Source: CAD feature listing. Evaluate the final solid. Frame: model axes, mm. A direction names the side the tool comes from. Give positions to 0.01 mm unless a question says otherwise; leave off trailing zeros. Write each loop counter-clockwise with the first axis right and the second up, starting at its lowest first coordinate (ties: lowest second). Pieces come first, ordered by that corner, then holes.
```python
from build123d import *

# Parameters (mm, degrees)
F0_W        = 3.9569679648
F0_H        = 9.3060303107
F0_R        = 0.75
F1_DEPTH    = 2
F2_R        = 3.6
F3_DEPTH    = 25
F4_T1_DEPTH = 2
F4_T3_DEPTH = 12


# Not quite as in the source:
# - a fillet or chamfer that OpenCascade refuses, or shapes differently, is made with other operations: its cross-section is extruded or revolved along the edge and cut away or added


with BuildPart() as f1:
    # F0 (on Top) → F1 (new body)
    with BuildSketch(Plane.XY):
        with Locations((-9.7150150687, 6.8534435891)):
            Rectangle(F0_W, F0_H)
        with Locations((-9.7150150687, 7.7160103247)):
            Circle(F0_R, mode=Mode.SUBTRACT)
        with Locations((-9.7150150687, 9.6662240103)):
            Circle(F0_R, mode=Mode.SUBTRACT)
        with BuildLine():
            ThreePointArc((-3.4285871837, -2.0602887962), (-3.9991430252, 0.0827953119), (-3.3403764321, 2.2004284337))
            Line((-3.3403764321, 2.2004284337), (-7.7365310863, 2.2004284337))
            Line((-7.7365310863, 2.2004284337), (-11.693499051, 2.2004284337))
            Line((-11.693499051, 2.2004284337), (-11.693499051, -2.0602887962))
            Line((-11.693499051, -2.0602887962), (-3.4285871837, -2.0602887962))
        make_face()
        with Locations((-9.7150150687, 0)):
            Circle(F0_R, mode=Mode.SUBTRACT)
        with BuildLine():
            Line((3.3403764321, -2.0602887962), (3.3403764321, 2.2004284337))
            ThreePointArc((3.3403764321, 2.2004284337), (0, 4), (-3.3403764321, 2.2004284337))
            Line((-3.3403764321, 2.2004284337), (-3.3403764321, -2.0602887962))
            Line((-3.3403764321, -2.0602887962), (-3.4285871837, -2.0602887962))
            ThreePointArc((-3.4285871837, -2.0602887962), (0, -4), (3.4285871837, -2.0602887962))
            Line((3.4285871837, -2.0602887962), (3.3403764321, -2.0602887962))
        make_face()
        with BuildLine():
            ThreePointArc((3.3403764321, 2.2004284337), (3.8315470588, 1.1485848405), (4, 0))
            ThreePointArc((4, 0), (3.8545005341, -1.06903023), (3.4285871837, -2.0602887962))
            Line((3.4285871837, -2.0602887962), (11.693499051, -2.0602887962))
            Line((11.693499051, -2.0602887962), (11.693499051, 2.2004284337))
            Line((11.693499051, 2.2004284337), (7.7365310863, 2.2004284337))
            Line((7.7365310863, 2.2004284337), (3.3403764321, 2.2004284337))
        make_face()
        with Locations((9.7150150687, 0)):
            Circle(F0_R, mode=Mode.SUBTRACT)
        with Locations((9.7150150687, 6.8534435891)):
            Rectangle(F0_W, F0_H)
        with Locations((9.7150150687, 7.7160103247)):
            Circle(F0_R, mode=Mode.SUBTRACT)
        with Locations((9.7150150687, 9.6662240103)):
            Circle(F0_R, mode=Mode.SUBTRACT)
        with BuildLine():
            Line((-3.3403764321, -2.0602887962), (-3.3403764321, 2.2004284337))
            ThreePointArc((-3.3403764321, 2.2004284337), (-3.9991430252, 0.0827953119), (-3.4285871837, -2.0602887962))
            Line((-3.4285871837, -2.0602887962), (-3.3403764321, -2.0602887962))
        make_face()
        with BuildLine():
            ThreePointArc((3.4285871837, -2.0602887962), (3.8545005341, -1.06903023), (4, 0))
            ThreePointArc((4, 0), (3.8315470588, 1.1485848405), (3.3403764321, 2.2004284337))
            Line((3.3403764321, 2.2004284337), (3.3403764321, -2.0602887962))
            Line((3.3403764321, -2.0602887962), (3.4285871837, -2.0602887962))
        make_face()
    extrude(amount=F1_DEPTH)

    # F2 (on face) → F3 (cut)
    with BuildSketch(Plane.XY.offset(2)):
        Circle(F2_R)
    extrude(amount=-F3_DEPTH, mode=Mode.SUBTRACT)

    # F4: fillet of radius 2 on 8 edges, made by hand

    # F4_s2 → F4_t1 (join)
    with BuildSketch(Plane.XY):
        with BuildLine():
            ThreePointArc((-7.7365310863, 4.2004284337), (-7.1507446486, 2.7862148714), (-5.7365310863, 2.2004284337))
            Line((-5.7365310863, 2.2004284337), (-7.7365310863, 2.2004284337))
            Line((-7.7365310863, 2.2004284337), (-7.7365310863, 4.2004284337))
        make_face()
        with BuildLine():
            ThreePointArc((5.7365310863, 2.2004284337), (7.1507446486, 2.7862148714), (7.7365310863, 4.2004284337))
            Line((7.7365310863, 4.2004284337), (7.7365310863, 2.2004284337))
            Line((7.7365310863, 2.2004284337), (5.7365310863, 2.2004284337))
        make_face()
    extrude(amount=F4_T1_DEPTH)

    # F4_s4 → F4_t3 (cut)
    with BuildSketch(Plane.XY.offset(-5)):
        with BuildLine():
            ThreePointArc((9.693499051, 11.5064587444), (11.1077126134, 10.9206723068), (11.693499051, 9.5064587444))
            Line((11.693499051, 9.5064587444), (11.693499051, 11.5064587444))
            Line((11.693499051, 11.5064587444), (9.693499051, 11.5064587444))
        make_face()
        with BuildLine():
            ThreePointArc((7.7365310863, 9.5064587444), (8.3223175239, 10.9206723068), (9.7365310863, 11.5064587444))
            Line((9.7365310863, 11.5064587444), (7.7365310863, 11.5064587444))
            Line((7.7365310863, 11.5064587444), (7.7365310863, 9.5064587444))
        make_face()
        with BuildLine():
            ThreePointArc((-7.7365310863, 9.5064587444), (-8.3223175239, 10.9206723068), (-9.7365310863, 11.5064587444))
            Line((-9.7365310863, 11.5064587444), (-7.7365310863, 11.5064587444))
            Line((-7.7365310863, 11.5064587444), (-7.7365310863, 9.5064587444))
        make_face()
        with BuildLine():
            ThreePointArc((-9.693499051, 11.5064587444), (-11.1077126134, 10.9206723068), (-11.693499051, 9.5064587444))
            Line((-11.693499051, 9.5064587444), (-11.693499051, 11.5064587444))
            Line((-11.693499051, 11.5064587444), (-9.693499051, 11.5064587444))
        make_face()
        with BuildLine():
            ThreePointArc((-11.693499051, -0.0602887962), (-11.1077126134, -1.4745023586), (-9.693499051, -2.0602887962))
            Line((-9.693499051, -2.0602887962), (-11.693499051, -2.0602887962))
            Line((-11.693499051, -2.0602887962), (-11.693499051, -0.0602887962))
        make_face()
        with BuildLine():
            ThreePointArc((9.693499051, -2.0602887962), (11.1077126134, -1.4745023586), (11.693499051, -0.0602887962))
            Line((11.693499051, -0.0602887962), (11.693499051, -2.0602887962))
            Line((11.693499051, -2.0602887962), (9.693499051, -2.0602887962))
        make_face()
    extrude(amount=F4_T3_DEPTH, mode=Mode.SUBTRACT)


solid = f1.part
```
1. Cut plane A-A, the plane x = 0. Return the cut outline in (y, z).
2. Line query: L1, parallel to X at y = 10, z = 0.8; L2, parallel to X at y = 6.25, z = 1.25; L3, parallel to Y at x = -5.25, z = 0.6. Output: solid intervals per line, ascending.
3. Access query for faces 1 (the cylindrical face through (-10.3, 9.2, 1)), 2 (the cylindrical face through (-8.3, 10.9, 1)), 3 (the flat face through (7, -2.06, 1)). Directions: +Z, -Z, +X, -X, +Y, -Y. A direction counts if a zero-diameter tool reaches every point of the face in a straight line with its end or side. Return the directions, or none.
4. Cut plane C-C, the plane x = -9.25. Return the cut outline in (y, z), then the cut area to 3 significant figures.
5. Cut plane D-D, the plane z = 0.9. Return the cut outline in (x, y).
6. Cut plane B-B, the plane y = -1. Return the cut outline in (x, z), then the cut area to 3 significant figures.
7. Contact query for flat-ended pins moving along their axis: P1, Ø0.9, axis at x = -9.72, y = 0, coming from the -Z side; P2, Ø1, axis at x = -4.5, z = 1, coming from the +Y side. Output: stop coordinate, or through.
8. Mould query, pull axis X, two halves, no side actions, for faces 4 (the cylindrical face through (0, -4, 1)), 5 (the cylindrical face through (8.3, 10.9, 1)), 6 (the cylindrical face through (-11.1, 10.93, 0.99)), 7 (the flat face through (5, 2, 2)). Classes: +X half, -X half, draft (parallel to the pull), parting line (faces both ways), or undercut.
Response values:
1. outline: (-4, 0) - (-3.6, 0) - (-3.6, 2) - (-4, 2) - close; (3.6, 0) - (4, 0) - (4, 2) - (3.6, 2) - close
2. L1: x = -11.63 to -10.39, -9.04 to -7.8, 7.8 to 9.04, 10.39 to 11.63
2. L2: x = -11.69 to -7.74, 7.74 to 11.69
2. L3: y = -2.06 to 2.2
3. face 1: +Z, -Z
3. face 2: +Z, -Z, +Y
3. face 3: +Z, -Z, +X, -Y
4. outline: (-2.06, 0) - (-0.59, 0) - (-0.59, 2) - (-2.06, 2) - close; (0.59, 0) - (7.13, 0) - (7.13, 2) - (0.59, 2) - close; (8.3, 0) - (9.08, 0) - (9.08, 2) - (8.3, 2) - close; (10.25, 0) - (11.45, 0) - (11.45, 2) - (10.25, 2) - close
4. area: 20.0 mm2
5. outline: (-11.69, -0.06) arc R2 ccw to (-9.69, -2.06) - (-3.43, -2.06) arc R4 ccw to (3.43, -2.06) - (9.69, -2.06) arc R2 ccw to (11.69, -0.06) - (11.69, 9.51) arc R2 ccw to (9.72, 11.51) arc R2 ccw to (7.74, 9.51) - (7.74, 4.2) arc R2 cw to (5.74, 2.2) - (3.34, 2.2) arc R4 ccw to (-3.34, 2.2) - (-5.74, 2.2) arc R2 cw to (-7.74, 4.2) - (-7.74, 9.51) arc R2 ccw to (-9.72, 11.51) arc R2 ccw to (-11.69, 9.51) - close; hole circle Ø1.5 at (-9.72, 0); hole circle Ø1.5 at (-9.72, 7.72); hole circle Ø1.5 at (-9.72, 9.67); hole circle Ø7.2 at (0, 0); hole circle Ø1.5 at (9.72, 0); hole circle Ø1.5 at (9.72, 7.72); hole circle Ø1.5 at (9.72, 9.67)
6. outline: (-11.46, 0) - (-3.46, 0) - (-3.46, 2) - (-11.46, 2) - close; (3.46, 0) - (11.46, 0) - (11.46, 2) - (3.46, 2) - close
6. area: 32.0 mm2
7. P1: passes through
7. P2: stops at y = 2.2
8. face 4: parting line
8. face 5: undercut
8. face 6: -X half
8. face 7: draft
